```python
from build123d import *

# Parameters (mm, degrees)
F0_W           = 334.6
F0_H           = 25.4
F1_DEPTH       = 50.8
F4_D           = 8.8
F4_DEPTH       = 23.1302
F4_TIP         = 2.6437867237
F4_ON_F2_D     = 8.8
F4_ON_F2_DEPTH = 23.1302
F4_ON_F2_TIP   = 2.6437867237
F5_SIZE        = 5.08
F7_D           = 8.5


# Not quite as in the source:
# - a feature names something its author has since deleted; it is built from what else it names


with BuildPart() as f1:
    # F0 (on Top) → F1 (new body)
    with BuildSketch(Plane.XY):
        with Locations((164.5870582715, 12.7)):
            Rectangle(F0_W, F0_H)
    extrude(amount=F1_DEPTH)

    # F4
    with Locations(Plane(origin=(-2.7129417285, 0, 0), x_dir=(0, -1, 0), z_dir=(-1, 0, 0))):
        with Locations((-12.7, 41.91), (-12.7, 8.89)):
            Hole(F4_D / 2, depth=F4_DEPTH)
            with Locations((0, 0, -(F4_DEPTH + F4_TIP / 2))):  # 118° drill point
                Cone(0, F4_D / 2, F4_TIP, mode=Mode.SUBTRACT)

    # F4 on F2
    with Locations(Plane.YZ.offset(331.8870582715)):
        with Locations((12.7, 41.91), (12.7, 8.89)):
            Hole(F4_ON_F2_D / 2, depth=F4_ON_F2_DEPTH)
            with Locations((0, 0, -(F4_ON_F2_DEPTH + F4_ON_F2_TIP / 2))):  # 118° drill point
                Cone(0, F4_ON_F2_D / 2, F4_ON_F2_TIP, mode=Mode.SUBTRACT)

    # F5
    f5_edges = [f1.edges().sort_by_distance(p)[0] for p in [
        (164.587058, 25.4, 0),
    ]]
    chamfer(f5_edges, length=F5_SIZE)

    # F7 (through all)
    with Locations(Plane(origin=(0, 0, 0), x_dir=(1, 0, 0), z_dir=(0, 0, -1))):
        with Locations((48.0870582715, -12.7), (281.0870582715, -12.7)):
            Hole(F7_D / 2)


solid = f1.part
```
Source: CAD feature listing. Evaluate the final solid. Frame: model axes, mm. A direction names the side the tool comes from. Give positions to 0.01 mm unless a question says otherwise; leave off trailing zeros. Use CSV: the item, a comma, the result in double quotes. Start each with the question number.
1. Draft query along X for faces 1 (the cylindrical face through (285.333, 12.513, 25.756)), 2 (the conical face through (306.57, 12.14, 9.41)), 3 (the cylindrical face through (9.014, 12.127, 46.273)). Return one class per face: +X half, -X half, draft (parallel to the pull), parting line (faces both ways), or undercut.
2. Ray query, L1, parallel to Z at x = 4.75, y = 12.7; L2, parallel to Z at x = 15, y = 9; L3, parallel to Y at x = 8, z = 41. Return the intervals inside material, ascending.
3. Pin query (flat end, axial travel): pin 1 (10 mm diameter, centred on y = 12.7, z = 8.89, fed in from +X); pin 2 (5.5 mm diameter, centred on y = 12.7, z = 41.91, fed in from +X); pin 3 (5 mm diameter, centred on y = 12.5, z = 41, fed in from -X); pin 4 (7 mm diameter, centred on y = 12.7, z = 8.89, fed in from +X). Return the tip coordinate at first contact, or that it passes through.
4. Reachability of faces 4 (the cylindrical face through (9.014, 8.304, 9.083)), 5 (the flat face through (-2.713, 13, 25)), 6 (the cylindrical face through (320.2, 8.5, 10.2)) from +Z, -Z, +X, -X, +Y, -Y: full face, straight path, thin tool, end or side. Return the list, or none.
Response:
1,face 1,"undercut"
1,face 2,"+X half"
1,face 3,"draft"
2,L1,"0 to 4.49, 13.29 to 37.51, 46.31 to 50.8"
2,L2,"0 to 6.51, 11.27 to 39.53, 44.29 to 50.8"
2,L3,"0 to 8.4, 17 to 25.4"
3,pin 1,"x = 331.89"
3,pin 2,"x = 307.77"
3,pin 3,"x = 21"
3,pin 4,"x = 308.22"
4,face 4,"-X"
4,face 5,"+Z, -Z, -X, +Y, -Y"
4,face 6,"+X"
